Can you work these out from the drawing? Everything is in mm from the part's minimum corner. A direction names the side the tool comes from. Give positions to 0.01 mm unless a question says otherwise; leave off trailing zeros. Write item = value, one per line. Start each with the question number.
1) On a 3-axis mill with a long thin cutter (end or side, diameter ignored), from which of +Z, -Z, +X, -X, +Y, -Y can I reach the whole of each face in a straight line? I mean the marked faces 1, 2 and 3. Say none if no direction works.
2) I need wall thicknesses on probe 1 along Y at (x, z) = (109, 55); probe 2 along X at (y, z) = (23.5, 7.5); probe 3 along X at (y, z) = (22, 16). Which ranges of each line are inside material? Lowest first, please. Write a range as from..to.
3) If we mould it in two halves opening along X, with no side actions, what happens to the marked faces 4, 5, 6 and 7? For each: +X half, -X half, draft (parallel to the pull), parting line (faces both ways), or undercut.
4) I'm going to push flat-ended pins straight in: pin 1 Ø15 at (x, z) = (63.5, 59.69) entering from -Y; pin 2 Ø5 at (x, y) = (122.5, 30.5) entering from +Z; pin 3 Ø15 at (x, z) = (19, 62.5) entering from -Y; pin 4 Ø9.5 at (x, y) = (40, 23) entering from +Z (1 decimal). Where does each tip first touch, or does it pass through?
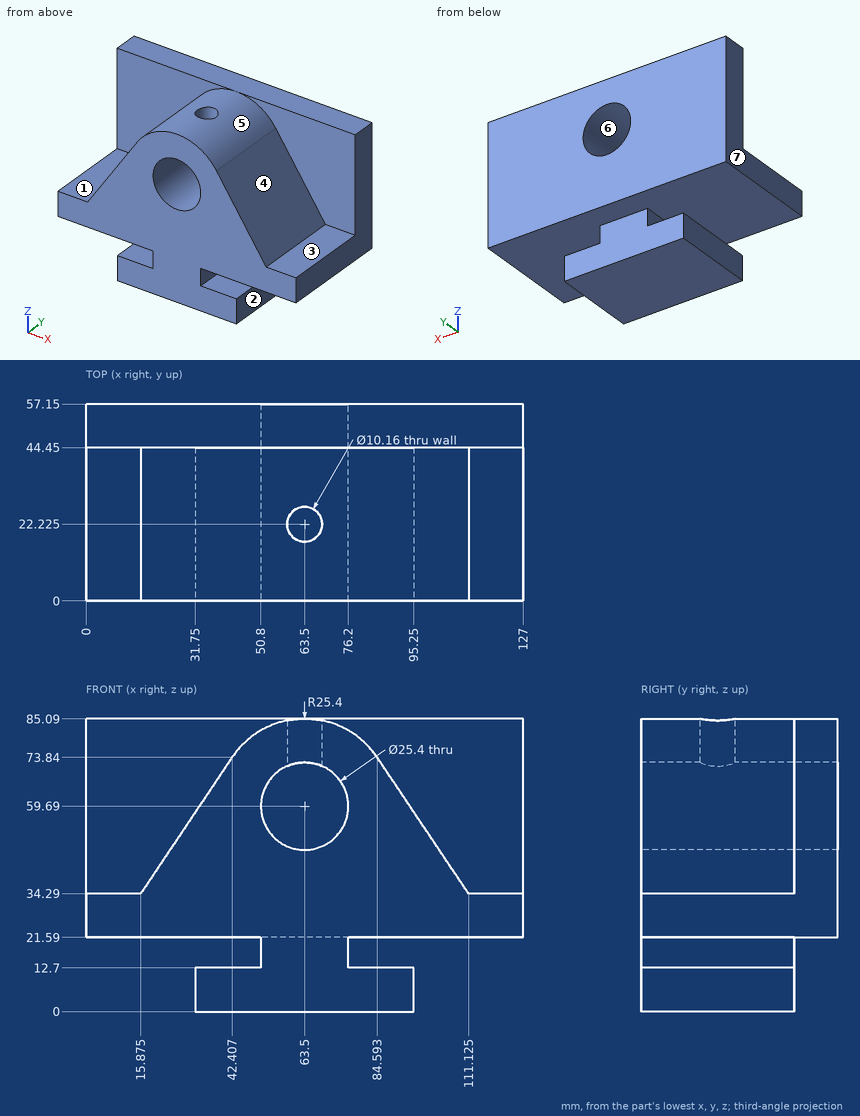
Answer list:
q1.face_1 = +Z, -X, -Y
q1.face_2 = -Z, +X, +Y, -Y
q1.face_3 = +Z, +X, -Y
q2.probe_1 = 44.45..57.15
q2.probe_2 = 31.75..95.25
q2.probe_3 = 50.8..76.2
q3.face_4 = +X half
q3.face_5 = parting line
q3.face_6 = undercut
q3.face_7 = -X half
q4.pin_1 = through
q4.pin_2 = 34.29
q4.pin_3 = 44.45
q4.pin_4 = 76.8
